from build123d import *

# Parameters (mm, degrees)
F1_DEPTH = 76.2
F2_W     = 50.8
F2_H     = 127
F3_DEPTH = 152.401
F4_R     = 38.1
F5_DEPTH = 25.401
F7_DEPTH = 25.401


with BuildPart() as f1:
    # F0 (on Front) → F1 (new body)
    with BuildSketch(Plane.XZ):
        Polygon((0, 34.412902), (0, 0), (101.6, 0), (101.6, 34.412902), (127, 34.412902), (127, 186.812902), (-25.4, 186.812902), (-25.4, 34.412902), align=None)
    extrude(amount=-F1_DEPTH)

    # F2 (on face) → F3 (cut, through all)
    with BuildSketch(Plane.YZ.offset(127)):
        with Locations((25.4, 123.312902)):
            Rectangle(F2_W, F2_H)
    extrude(amount=-F3_DEPTH, mode=Mode.SUBTRACT)

    # F4 (on face) → F5 (cut, through all)
    with BuildSketch(Plane.XZ.offset(-50.8)):
        with Locations((50.8, 110.612902)):
            Circle(F4_R)
    extrude(amount=-F5_DEPTH, mode=Mode.SUBTRACT)

    # F6 (on face) → F7 (cut, through all)
    with BuildSketch(Plane.XZ.offset(-50.8)):
        with BuildLine():
            Line((50.8, 186.812902), (-25.4, 186.812902))
            Line((-25.4, 186.812902), (-25.4, 110.612902))
            ThreePointArc((-25.4, 110.612902), (-3.081537, 164.494439), (50.8, 186.812902))
        make_face()
        with BuildLine():
            Line((127, 186.812902), (50.8, 186.812902))
            ThreePointArc((50.8, 186.812902), (104.681537, 164.494439), (127, 110.612902))
            Line((127, 110.612902), (127, 186.812902))
        make_face()
    extrude(amount=-F7_DEPTH, mode=Mode.SUBTRACT)


solid = f1.part
Can you work these out from the model? Positions are in its coordinate system, mm. A direction names the side the tool comes from. Round coordinates to 2 decimals unless told otherwise and drop trailing zeros. Order: outer loops, then holes, each group sorted by start corner. A loop starts at its lowest first (then second) coordinate and runs counter-clockwise, first axis right, second up. Notation, with made-up numbers: (-26, 62.25) - (-19, 62.25) arc R33 ccw to (-19, 95.25) - close; hole circle Ø8 at (-17, 12). An arc over 180 degrees is marked (long way). Answer in a Markdown table with one row per item.
(1) Which directions (+Z, -Z, +X, -X, +Y, -Y) give clear straight access to the entire face, cutting with the end or side of a thin tool? Please do faces 1 (the face through (50, 38, 0)), 2 (the face through (-13, 38, 34.413)), 3 (the face through (52, 50.8, 151)).
From the geometry:
| item | result |
|---|---|
| face 1 | -Z, +X, -X, +Y, -Y |
| face 2 | -Z, -X, +Y, -Y |
| face 3 | +Z, +X, -X, -Y |
(2) Suppose I cut it at A-A, the plane y = 62.5. Please give me the cut outline in (x, z), plus the area to 3 significant figures.
From the geometry:
| item | result |
|---|---|
| outline | (-25.4, 34.41) - (0, 34.41) - (0, 0) - (101.6, 0) - (101.6, 34.41) - (127, 34.41) - (127, 110.61) arc R76.2 ccw to (50.8, 186.81) arc R76.2 ccw to (-25.4, 110.61) - close; hole circle Ø76.2 at (50.8, 110.61) |
| area | 19,700 mm2 |
(3) Please list where these lines run through material, in increasing order: L1, parallel to Z at x = 50.8, y = 69; L2, parallel to Y at x = -12, z = 74; L3, parallel to X at y = 68.5, z = 122.5. Write a range as from..to.
From the geometry:
| item | result |
|---|---|
| L1 | z = 0..72.51, 148.71..186.81 |
| L2 | y = 50.8..76.2 |
| L3 | x = -24.47..14.6, 87..126.07 |
(4) Suppose I cut it at B-B, the plane z = 91.5. Please give me the cut outline in (x, y), plus the area to 3 significant figures.
From the geometry:
| item | result |
|---|---|
| outline | (-25.4, 50.8) - (17.84, 50.8) - (17.84, 76.2) - (-25.4, 76.2) - close; (83.76, 50.8) - (127, 50.8) - (127, 76.2) - (83.76, 76.2) - close |
| area | 2,200 mm2 |
(5) For P1, Ø2, axis at x = 28.5, y = 51, coming from the +Z side; P2, Ø3, axis at x = 89, y = 67.5, coming from the +Z side; P3, Ø1.5, axis at x = 76, y = 42.5, coming from the -Z side; P4, Ø10.5, axis at y = 47, z = 24.5, coming from the -X side, each with a flat end and sliding along its axis, tell me the tip position at first contact or that it passes through.
From the geometry:
| item | result |
|---|---|
| P1 | stops at z = 183.78 |
| P2 | stops at z = 177.39 |
| P3 | stops at z = 0 |
| P4 | stops at x = 0 |
(6) If we mould it in two halves opening along Z, with no side actions, what happens to faces 4 (the face through (42.54, 63.32, 73.42)), 5 (the face through (101.6, 38, 17)), 6 (the face through (114, 38, 34.413)), 7 (the face through (52, 25, 59.813))? For each: released by +Z, released by -Z, zero draft, split by the parting line, or undercut.
From the geometry:
| item | result |
|---|---|
| face 4 | undercut |
| face 5 | zero draft |
| face 6 | released by -Z |
| face 7 | released by +Z |
(7) Suppose I cut it at C-C, the plane x = 35. Please give me the cut outline in (y, z).
From the geometry:
| item | result |
|---|---|
| outline | (0, 0) - (76.2, 0) - (76.2, 75.94) - (50.8, 75.94) - (50.8, 59.81) - (0, 59.81) - close; (50.8, 145.28) - (76.2, 145.28) - (76.2, 185.16) - (50.8, 185.16) - close |
(8) Suppose I cut it at D-D, the plane y = 16. Please give me the cut outline in (x, z).
From the geometry:
| item | result |
|---|---|
| outline | (-25.4, 34.41) - (0, 34.41) - (0, 0) - (101.6, 0) - (101.6, 34.41) - (127, 34.41) - (127, 59.81) - (-25.4, 59.81) - close |
